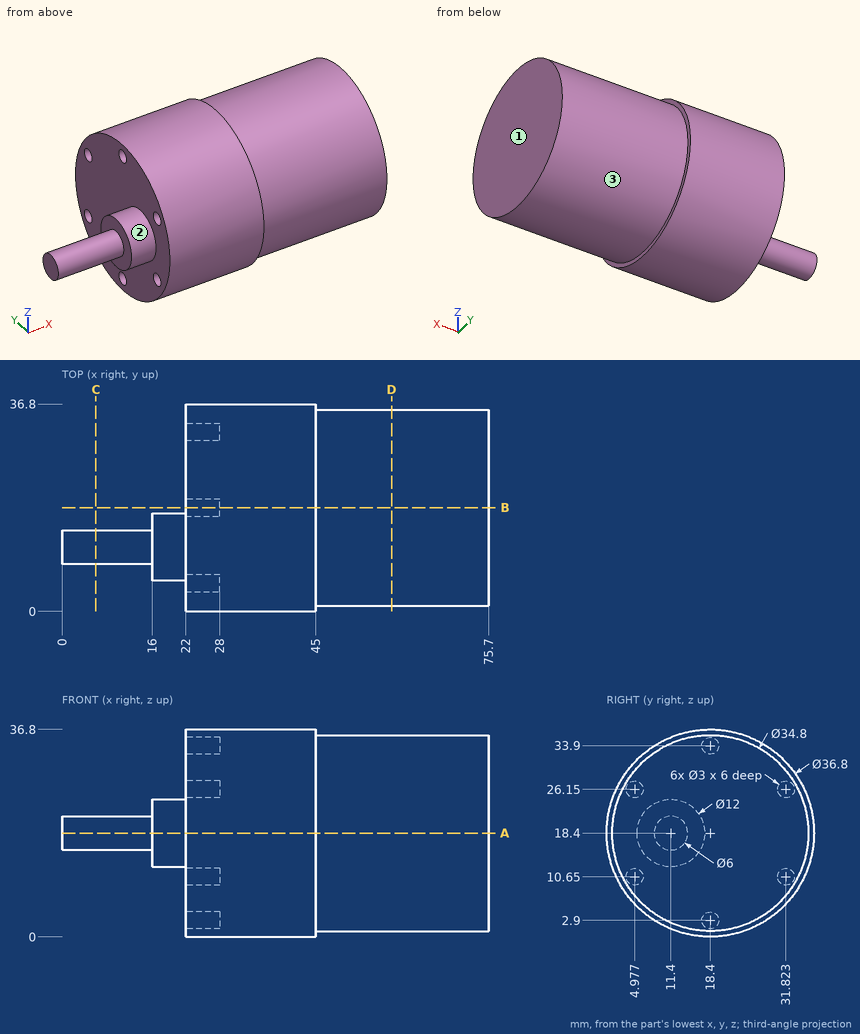
Print and shaded views of the part. All mm, measured from the part's lowest x, y and z. A direction names the side the tool comes from. Round coordinates to 2 decimals unless told otherwise and drop trailing zeros. Order: outer loops, then holes, each group sorted by start corner. A loop starts at its lowest first (then second) coordinate and runs counter-clockwise, first axis right, second up. Notation, with made-up numbers: (-37.5, 54) - (-29.5, 54) arc R18 cw to (-29.5, 85) - close; hole circle Ø7 at (29, -32.75). An arc over 180 degrees is marked (long way). Use a Markdown table: item, result.
1) Saw through at B-B on y = 18.4. Write the cut outline in (x, z).
Recorded:
| item | result |
|---|---|
| outline | (22, 0) - (45, 0) - (45, 1) - (75.7, 1) - (75.7, 35.8) - (45, 35.8) - (45, 36.8) - (22, 36.8) - (22, 35.4) - (28, 35.4) - (28, 32.4) - (22, 32.4) - (22, 4.4) - (28, 4.4) - (28, 1.4) - (22, 1.4) - close |
2) Saw through at A-A on z = 18.4. Write the cut outline in (x, y).
Recorded:
| item | result |
|---|---|
| outline | (0, 8.4) - (16, 8.4) - (16, 5.4) - (22, 5.4) - (22, 0) - (45, 0) - (45, 1) - (75.7, 1) - (75.7, 35.8) - (45, 35.8) - (45, 36.8) - (22, 36.8) - (22, 17.4) - (16, 17.4) - (16, 14.4) - (0, 14.4) - close |
3) Wall check: L1, parallel to Z at x = 24.25, y = 18.4; L2, parallel to Z at x = 23, y = 32 (1 decimal); L3, parallel to Y at x = 26, z = 10 (1 decimal). Give the ranges that are in metal, low to high.
Recorded:
| item | result |
|---|---|
| L1 | z = 0 to 1.4, 4.4 to 32.4, 35.4 to 36.8 |
| L2 | z = 6 to 9.2, 12.1 to 24.7, 27.6 to 30.8 |
| L3 | y = 2 to 3.6, 6.3 to 30.5, 33.2 to 34.8 |
4) Saw through at C-C on x = 6. Write the cut outline in (y, z).
Recorded:
| item | result |
|---|---|
| outline | circle Ø6 at (11.4, 18.4) |
5) Saw through at D-D on x = 58.5. Write the cut outline in (y, z), and give its area (3 significant figures).
Recorded:
| item | result |
|---|---|
| outline | circle Ø34.8 at (18.4, 18.4) |
| area | 951 mm² |
6) Tool access for the marked faces 1, 2 and 3: list every direction of +Z, -Z, +X, -X, +Y, -Y with a clear straight run to the whole face (end or side of a thin tool).
Recorded:
| item | result |
|---|---|
| face 1 | +Z, -Z, +X, +Y, -Y |
| face 2 | -X |
| face 3 | +X |
7) Flat gauge pins, fed straight in: pin 1 Ø8 at (x, z) = (18.5, 10.5) entering from -Y; pin 2 Ø3.5 at (y, z) = (5.5, 26) entering from -X; pin 3 Ø2 at (x, y) = (60, 7.5) entering from +Z. Where does each tip first touch, or does it go through?
Recorded:
| item | result |
|---|---|
| pin 1 | stops at y = 0.99 |
| pin 2 | stops at x = 22 |
| pin 3 | stops at z = 32.71 |
